Source: CAD feature listing. Evaluate the final solid. Frame: model axes, mm. Face numbers are marked on the shaded views. A direction names the side the tool comes from. Round coordinates to 2 decimals unless told otherwise and drop trailing zeros. Loops run counter-clockwise (first coordinate to the right, second up) from the corner with the lowest first, then second, coordinate; pieces in that order, holes last. Notation, with made-up numbers: M -35.75,30.25 L 2.25,30.25 A16 cw 2.25,56.25 Z; hole C 73.25,-12.5 d9. An arc over 180 degrees is marked long. One line per item, written item: value.
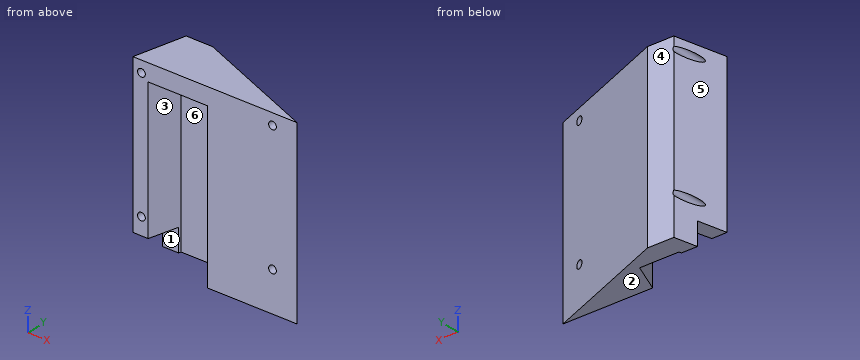
from build123d import *

# Parameters (mm, degrees)
EXTRUDE_1_DEPTH     = 63
EXTRUDE_2_DEPTH     = 6
SKETCH_3_W          = 8
SKETCH_3_H          = 10
CUT_EXTRUDE_1_DEPTH = 19
SKETCH_4_R          = 1.35
CUT_EXTRUDE_2_DEPTH = 27


with BuildPart() as part:
    # 草图1 → 凸台-拉伸1 (new body)
    with BuildSketch(Plane.XY):
        Polygon((5.368916437, 0), (10.737832874, 0), (13.433272115, 10.825245017), (27.262006405, 10.825245017), (31.5, 0), (63, 0), (18.696157585, 17.96451652), (9.426538108, 17.96451652), align=None)
    extrude(amount=EXTRUDE_1_DEPTH)

    # 草图2 → 凸台-拉伸2 (add)
    with BuildSketch(Plane.XY.offset(63)):
        Polygon((10.737832874, 0), (31.5, 0), (27.262006405, 10.825245017), (13.433272115, 10.825245017), align=None)
    extrude(amount=-EXTRUDE_2_DEPTH)

    # 草图3 → 切除-拉伸1 (cut)
    with BuildSketch(Plane(origin=(0, 0, 0), x_dir=(0, 0, -1), z_dir=(1, 0, 0))):
        with Locations((-4, 5)):
            Rectangle(SKETCH_3_W, SKETCH_3_H)
    extrude(amount=CUT_EXTRUDE_1_DEPTH, mode=Mode.SUBTRACT)

    # 草图4 → 切除-拉伸2 (cut)
    with BuildSketch(Plane.XZ):
        with Locations(Location((8.368916437, 59, 0), (0, 0, 270))):
            Circle(SKETCH_4_R)
        with Locations(Location((54.368916437, 59, 0), (0, 0, 270))):
            Circle(SKETCH_4_R)
        with Locations(Location((54.368916437, 14, 0), (0, 0, 270))):
            Circle(SKETCH_4_R)
        with Locations(Location((8.368916437, 14, 0), (0, 0, 270))):
            Circle(SKETCH_4_R)
    extrude(amount=-CUT_EXTRUDE_2_DEPTH, mode=Mode.SUBTRACT)


solid = part.part
1. Section query B-B (y = 1.5). Return the cut outline in (x, z).
Report:
outline: M 5.71,8 L 11.11,8 L 11.11,57 L 30.91,57 L 30.91,0 L 59.3,0 L 59.3,63 L 5.71,63 Z; hole C 8.37,14 d2.7; hole C 8.37,59 d2.7; hole C 54.37,14 d2.7; hole C 54.37,59 d2.7
2. Pull-direction query (X, two-part tool) for the marked faces 4, 5 and 6; classes: released by +X, released by -X, zero draft, split by the parting line, or undercut.
Report:
face 4: zero draft
face 5: released by -X
face 6: undercut
3. Section query D-D (x = 12). Return the cut outline in (y, z).
Report:
outline: M 0,57 L 5.07,57 L 5.07,8 L 10,8 L 10,0 L 17.96,0 L 17.96,63 L 0,63 Z
4. Pin query (flat end, axial travel): pin 1 (6 mm diameter, centred on y = 5.5, z = 19.5, fed in from +X); pin 2 (4 mm diameter, centred on y = 10.5, z = 49.5, fed in from +X); pin 3 (3 mm diameter, centred on x = 54.37, z = 14, fed in from +Y). Return the tip coordinate at first contact, or that it passes through.
Report:
pin 1: stops at x = 56.83
pin 2: stops at x = 42.04
pin 3: stops at y = 4.11
5. Section query C-C (z = 14). Return the cut outline in (x, y).
Report:
outline: M 5.37,0 L 7.02,0 L 7.02,7.31 Z; M 9.72,0 L 10.74,0 L 13.43,10.83 L 27.26,10.83 L 31.5,0 L 53.02,0 L 53.02,4.05 L 18.7,17.96 L 9.72,17.96 Z; M 55.72,0 L 63,0 L 55.72,2.95 Z
6. Ray query, line 1 (X direction, y = 1.3, z = 59); line 2 (X direction, y = 1.2, z = 59); line 3 (X direction, y = 1.5, z = 14). Return the intervals inside material, ascending. Write a range as [from, to].
Report:
line 1: x = [5.66, 7.02], [9.72, 53.02], [55.72, 59.79]
line 2: x = [5.64, 7.02], [9.72, 53.02], [55.72, 60.04]
line 3: x = [5.71, 7.02], [9.72, 11.11], [30.91, 53.02], [55.72, 59.3]
7. Reachability of the marked faces 1, 2 and 3 from +Z, -Z, +X, -X, +Y, -Y: full face, straight path, thin tool, end or side. Return the list, or none.
Report:
face 1: -Z, -X, -Y
face 2: -Z, +X, -X, +Y, -Y
face 3: -Z, -Y
8. Section query A-A (z = 53.5). Return the cut outline in (x, y), and give its area (3 significant figures).
Report:
outline: M 5.37,0 L 10.74,0 L 13.43,10.83 L 27.26,10.83 L 31.5,0 L 63,0 L 18.7,17.96 L 9.43,17.96 Z
area: 414 mm2
